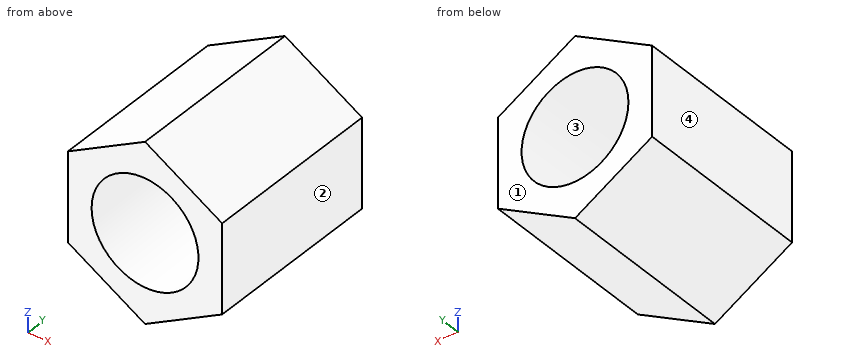
Autodesk Inventor part; units mm, degrees
ref_plane "YZ Plane" through (0, 0, 0) normal (1, 0, 0) x (0, 1, 0)
ref_plane "XZ Plane" through (0, 0, 0) normal (0, 1, 0) x (-1, 0, 0)
ref_plane "XY Plane" through (0, 0, 0) normal (0, 0, 1) x (1, 0, 0)
sketch "Эскиз1" plane through (0, 0, 0) normal (0, 1, 0) x (-1, 0, 0)
  line L0 (0, 3.5153) -> (0, -1.4847)
  line L1 (0, -1.4847) -> (-2.1651, -0.2347)
  line L2 (-2.1651, -0.2347) -> (-2.1651, 2.2653)
  line L3 (-2.1651, 2.2653) -> (0, 3.5153)
  line L4 (0, 3.5153) -> (2.1651, 2.2653)
  line L5 (2.1651, 2.2653) -> (2.1651, -0.2347)
  line L6 (2.1651, -0.2347) -> (0, -1.4847)
  circle A0 centre (0, 1.0153) radius 1.5
  point P0 (0, 0)
  dimension "d0" = 5
  dimension "d1" = 3
extrude "Выдавливание1" add sketch "Эскиз1" along normal blind 5 contours L4 L5 L6 L0 A0 | L0 A0 L1 L2 L3
thread "Резьба1"
properties part number "rack_05"
The model under review builds one solid part; all positions refer to its coordinate system, in mm. Face numbers are marked on the shaded views. Coordinates: 2 decimals unless noted, no trailing zeros. Write each loop counter-clockwise with the first axis right and the second up, starting at its lowest first coordinate (ties: lowest second). Pieces come first, ordered by that corner, then holes. Notation, with made-up numbers: M 68.5,79 L 111.5,79 A26 cw 111.5,99 Z; hole C 39,12.5 d7. An arc over 180 degrees is marked long. Put each result on its own line as item: value.
1) Add section B-B on x = -0.6. Give the boundary of the cut face in (y, z).
Computed:
outline: M 0,-1.14 L 5,-1.14 L 5,-0.36 L 0,-0.36 Z; M 0,2.39 L 5,2.39 L 5,3.17 L 0,3.17 Z
2) Add section A-A on z = 0.2. Give the boundary of the cut face in (x, y).
Computed:
outline: M -2.17,0 L -1.26,0 L -1.26,5 L -2.17,5 Z; M 1.26,0 L 2.17,0 L 2.17,5 L 1.26,5 Z
3) Clearance check with flat-ended pins moving along their axes: pin 1 Ø1.8 at (x, z) = (0, 1.02) entering from +Y; pin 2 Ø1.5 at (x, y) = (-1, 3) entering from +Z. State where each tip first meets the part, or that it passes through.
Computed:
pin 1: passes through
pin 2: stops at z = 3.37
4) Draft analysis for pull direction X (two halves, no side actions). For the marked faces 1, 2, 3 and 4, state which applies: released by +X, released by -X, zero draft, split by the parting line, or undercut.
Computed:
face 1: zero draft
face 2: released by +X
face 3: undercut
face 4: released by -X
5) Wall thickness on probe 1 along Z at (x, y) = (-1.15, 3.55); probe 2 along X at (y, z) = (4.15, -0.2); probe 3 along X at (y, z) = (3.85, 1.5): over which ranges is each line inside the solid? List them lowest first. Write a range as [from, to].
Computed:
probe 1: z = [-0.82, 0.05], [1.98, 2.85]
probe 2: x = [-2.17, -0.88], [0.88, 2.17]
probe 3: x = [-2.17, -1.42], [1.42, 2.17]
6) Add section D-D on z = -1.1. Give the boundary of the cut face in (x, y).
Computed:
outline: M -0.67,0 L 0.67,0 L 0.67,5 L -0.67,5 Z
7) Add section C-C on y = 2.75. Give the boundary of the cut face in (x, z), then the cut area to 3 significant figures.
Computed:
outline: M -2.17,-0.23 L 0,-1.48 L 2.17,-0.23 L 2.17,2.27 L 0,3.52 L -2.17,2.27 Z; hole C 0,1.02 d3
area: 9.17 mm2
